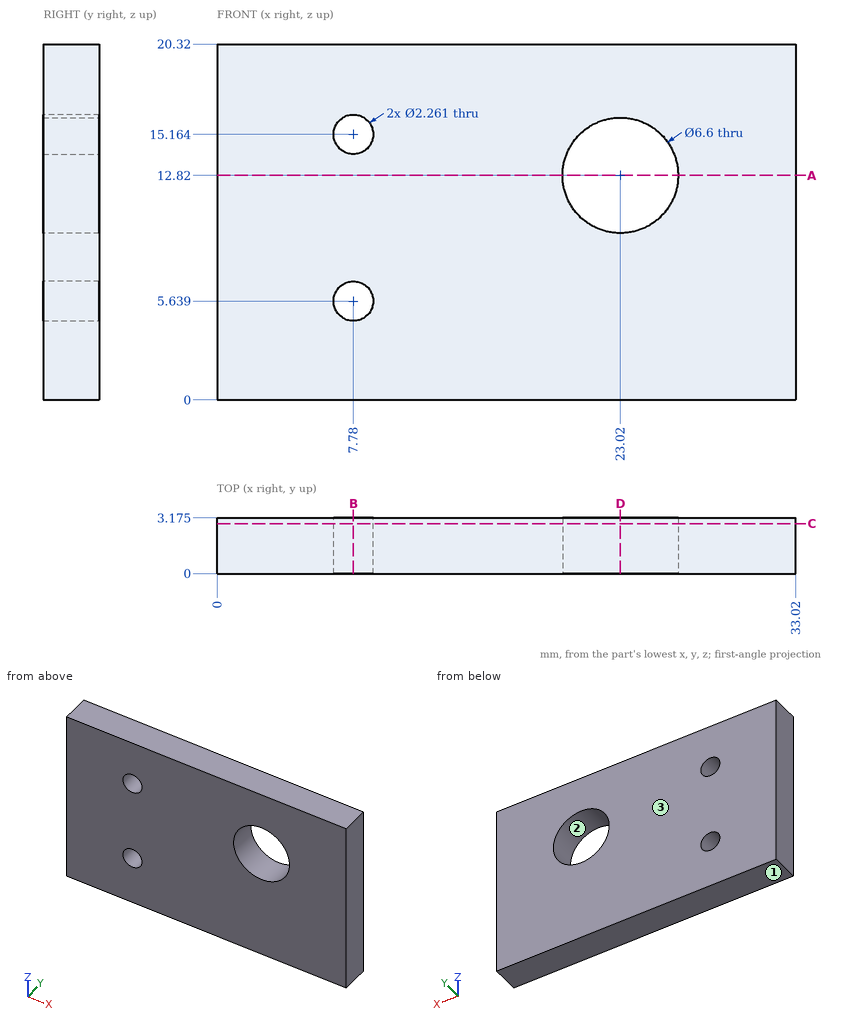
The drawing under review shows one solid part. Ordinate dimensions are in mm from its lowest x, y, z. Coordinates: 2 decimals unless noted, no trailing zeros. Order: outer loops, then holes, each group sorted by start corner. A loop starts at its lowest first (then second) coordinate and runs counter-clockwise, first axis right, second up. Notation, with made-up numbers: (0.25, -21.75) -> (56.25, -21.75) arc R20 ccw to (56.25, 3.25) -> close; hole circle Ø4 at (30.5, 12). An arc over 180 degrees is marked (long way). Use CSV: the item, a comma, the result in double quotes. Start each with the question number.
Item 1: Draft analysis for pull direction Z (two halves, no side actions). For the marked faces 1, 2 and 3, state which applies: pulls with the +Z half, pulls with the -Z half, needs draft (parallel to the pull), parting line crosses it, or undercut.
Item 2: We need section C-C, the plane y = 2.85. Give the boundary of the cut face in (x, z), then the cut area to 3 significant figures.
Item 3: We need section A-A, the plane z = 12.82. Give the boundary of the cut face in (x, y) (1 decimal).
Item 4: Wall thickness on probe 1 along X at (y, z) = (1.7, 15); probe 2 along Z at (x, y) = (7, 0.5) (1 decimal); probe 3 along X at (y, z) = (2.45, 12.82): over which ranges is each line inside the solid? List them lowest first.
Item 5: We need section B-B, the plane x = 7.78. Give the boundary of the cut face in (y, z) (1 decimal).
Item 6: We need section D-D, the plane x = 23.02. Give the boundary of the cut face in (y, z) (1 decimal).
Derived:
1,face 1,"pulls with the -Z half"
1,face 2,"undercut"
1,face 3,"needs draft"
2,outline,"(0, 0) -> (33.02, 0) -> (33.02, 20.32) -> (0, 20.32) -> close; hole circle Ø2.26 at (7.78, 5.64); hole circle Ø2.26 at (7.78, 15.16); hole circle Ø6.6 at (23.02, 12.82)"
2,area,"629 mm^2"
3,outline,"(0, 0) -> (19.7, 0) -> (19.7, 3.2) -> (0, 3.2) -> close; (26.3, 0) -> (33, 0) -> (33, 3.2) -> (26.3, 3.2) -> close"
4,probe 1,"x = 0 to 6.66, 8.9 to 20.54, 25.5 to 33.02"
4,probe 2,"z = 0 to 4.8, 6.5 to 14.3, 16 to 20.3"
4,probe 3,"x = 0 to 19.72, 26.32 to 33.02"
5,outline,"(0, 0) -> (3.2, 0) -> (3.2, 4.5) -> (0, 4.5) -> close; (0, 6.8) -> (3.2, 6.8) -> (3.2, 14) -> (0, 14) -> close; (0, 16.3) -> (3.2, 16.3) -> (3.2, 20.3) -> (0, 20.3) -> close"
6,outline,"(0, 0) -> (3.2, 0) -> (3.2, 9.5) -> (0, 9.5) -> close; (0, 16.1) -> (3.2, 16.1) -> (3.2, 20.3) -> (0, 20.3) -> close"
